```python
from build123d import *

# Parameters (mm, degrees)
Y_KSEKLIK_EKSTR_ZYON1_DEPTH = 7
IZIM2_R                     = 1.5
KES_EKSTR_ZYON1_DEPTH       = 7
PAH1_SIZE                   = 2.5
IZIM3_R                     = 2
KES_EKSTR_ZYON2_DEPTH       = 10
KES_EKSTR_ZYON3_START       = -10
IZIM4_R                     = 2
KES_EKSTR_ZYON3_DEPTH       = 10
RADYUS1_R                   = 20
IZIM5_W                     = 90
IZIM5_H                     = 10
IZIM5_W_2                   = 10
IZIM5_H_2                   = 70
KES_EKSTR_ZYON4_DEPTH       = 10
RADYUS2_R                   = 4
KES_EKSTR_ZYON5_DEPTH       = 10
IZIM8_W                     = 5
IZIM8_H                     = 53
KES_EKSTR_ZYON6_DEPTH       = 10
IZIM9_W                     = 8.724341423
IZIM9_H                     = 2.178581573
IZIM9_W_2                   = 9.164333206
Y_KSEKLIK_EKSTR_ZYON2_DEPTH = 10
IZIM10_W                    = 140
IZIM10_H                    = 10
KES_EKSTR_ZYON7_DEPTH       = 10
IZIM11_W                    = 10
IZIM11_H                    = 4
Y_KSEKLIK_EKSTR_ZYON3_DEPTH = 7
RADYUS3_R                   = 10
IZIM12_W                    = 4
IZIM12_H                    = 9
Y_KSEKLIK_EKSTR_ZYON4_DEPTH = 7
RADYUS4_R                   = 4
IZIM13_R                    = 1.5
KES_EKSTR_ZYON8_DEPTH       = 7
PAH2_SIZE                   = 1.5
RADYUS5_R                   = 2
IZIM14_W                    = 144.535934645
IZIM14_H                    = 70
KES_EKSTR_ZYON9_DEPTH       = 2
RADYUS6_R                   = 2
KES_EKSTR_ZYON10_DEPTH      = 5
KES_EKSTR_ZYON10_DEPTH_BACK = 5
IZIM15_R                    = 7.5
IZIM16_R                    = 1.75
KES_EKSTR_ZYON11_DEPTH      = 7
IZIM17_R                    = 1.75
KES_EKSTR_ZYON12_DEPTH      = 10
Y_KSEKLIK_EKSTR_ZYON5_START = -5
IZIM18_R                    = 3
IZIM18_R_2                  = 2
Y_KSEKLIK_EKSTR_ZYON5_DEPTH = 5
IZIM19_W                    = 4
IZIM19_H                    = 10
KES_EKSTR_ZYON13_DEPTH      = 10


# Some blends are built 0.0001 mm under size
with BuildPart() as part:
    # izim1 → Y_kseklik-Ekstr_zyon1 (new body)
    with BuildSketch(Plane(origin=(0, 0, 0), x_dir=(1, 0, 0), z_dir=(0, 1, 0))):
        Polygon((0, 0), (0, 53), (15, 53), (30, 66.5), (150, 66.5), (150, -13.5), (30, -13.5), (15, 0), align=None)
    extrude(amount=Y_KSEKLIK_EKSTR_ZYON1_DEPTH)

    # izim2 → Kes-Ekstr_zyon1 (cut)
    with BuildSketch(Plane(origin=(0, 7, 0), x_dir=(1, 0, 0), z_dir=(0, 1, 0))):
        with Locations(Location((2.5, 41.25, 0), (0, 0, 270))):
            Circle(IZIM2_R)
        with Locations(Location((2.5, 11.75, 0), (0, 0, 270))):
            Circle(IZIM2_R)
    extrude(amount=-KES_EKSTR_ZYON1_DEPTH, mode=Mode.SUBTRACT)

    # Pah1
    # the kernel refuses this chamfer: 2.5 mm, written as the material it takes off along each edge
    with BuildSketch(Plane(origin=(2.5, 7, -41.25), x_dir=(0, 0, 1), z_dir=(-1, 0, 0))) as pah1_piece_1:
        Polygon((1.5 + PAH1_SIZE, 0), (1.5, -PAH1_SIZE), (1.5, 0), align=None)
    revolve(axis=Axis((2.5, 7, -41.25), (0, 1, 0)), mode=Mode.SUBTRACT)
    with BuildSketch(Plane(origin=(2.5, 7, -11.75), x_dir=(0, 0, 1), z_dir=(-1, 0, 0))) as pah1_piece_2:
        Polygon((1.5 + PAH1_SIZE, 0), (1.5, -PAH1_SIZE), (1.5, 0), align=None)
    revolve(axis=Axis((2.5, 7, -11.75), (0, 1, 0)), mode=Mode.SUBTRACT)

    # izim3 → Kes-Ekstr_zyon2 (cut)
    with BuildSketch(Plane.XY.offset(13.5)):
        with Locations((46.24, 3.5)):
            Circle(IZIM3_R)
    extrude(amount=-KES_EKSTR_ZYON2_DEPTH, mode=Mode.SUBTRACT)

    # izim4 → Kes-Ekstr_zyon3 (cut)
    with BuildSketch(Plane(origin=(0, 0, -66.5), x_dir=(-1, 0, 0), z_dir=(0, 0, -1)).offset(KES_EKSTR_ZYON3_START)):
        with Locations(Location((-46.24, 3.5, 0), (0, 0, 180))):
            Circle(IZIM4_R)
    extrude(amount=KES_EKSTR_ZYON3_DEPTH, mode=Mode.SUBTRACT)

    # Radyus1
    radyus1_edges = [part.edges().sort_by_distance(p)[0] for p in [
        (150, 3.5, -66.5),
        (150, 3.5, 13.5),
    ]]
    fillet(radyus1_edges, radius=RADYUS1_R)

    # izim5 → Kes-Ekstr_zyon4 (cut)
    with BuildSketch(Plane(origin=(0, 7, 0), x_dir=(1, 0, 0), z_dir=(0, 1, 0))):
        with Locations((75, -3.5)):
            Rectangle(IZIM5_W, IZIM5_H)
        with Locations((75, 26.5)):
            Rectangle(IZIM5_W, IZIM5_H)
        with Locations((75, 41.5)):
            Rectangle(IZIM5_W, IZIM5_H)
        with Locations((75, 56.5)):
            Rectangle(IZIM5_W, IZIM5_H)
        with Locations((75, 11.5)):
            Rectangle(IZIM5_W, IZIM5_H)
        with Locations((130, 26.5)):
            Rectangle(IZIM5_W_2, IZIM5_H_2)
    extrude(amount=-KES_EKSTR_ZYON4_DEPTH, mode=Mode.SUBTRACT)

    # Radyus2
    radyus2_edges = [part.edges().sort_by_distance(p)[0] for p in [
        (135, 3.5, -61.5),
        (135, 3.5, 8.5),
    ]]
    fillet(radyus2_edges, radius=RADYUS2_R)

    # izim6 → Kes-Ekstr_zyon5 (cut)
    with BuildSketch(Plane(origin=(0, 7, 0), x_dir=(1, 0, 0), z_dir=(0, 1, 0))):
        with BuildLine():
            Line((139, -6), (139, 59))
            ThreePointArc((139, 59), (143.530979443, 53.484870133), (145, 46.5))
            Line((145, 46.5), (145, 6.5))
            ThreePointArc((145, 6.5), (143.530979443, -0.484870133), (139, -6))
        make_face()
    extrude(amount=-KES_EKSTR_ZYON5_DEPTH, mode=Mode.SUBTRACT)

    # izim8 → Kes-Ekstr_zyon6 (cut)
    with BuildSketch(Plane(origin=(0, 7, 0), x_dir=(1, 0, 0), z_dir=(0, 1, 0))):
        with Locations((2.5, 26.5)):
            Rectangle(IZIM8_W, IZIM8_H)
    extrude(amount=-KES_EKSTR_ZYON6_DEPTH, mode=Mode.SUBTRACT)

    # izim9 → Y_kseklik-Ekstr_zyon2 (add)
    with BuildSketch(Plane.ZY.offset(-5)):
        with Locations((-12.430411948, 5.910709214)):
            Rectangle(IZIM9_W, IZIM9_H)
        with Locations((-41.247168871, 5.910709214)):
            Rectangle(IZIM9_W_2, IZIM9_H)
    extrude(amount=-Y_KSEKLIK_EKSTR_ZYON2_DEPTH)

    # izim10 → Kes-Ekstr_zyon7 (cut)
    with BuildSketch(Plane(origin=(0, 7, 0), x_dir=(1, 0, 0), z_dir=(0, 1, 0))):
        with Locations((85, -13.5)):
            Rectangle(IZIM10_W, IZIM10_H)
        with Locations((85, 66.5)):
            Rectangle(IZIM10_W, IZIM10_H)
    extrude(amount=-KES_EKSTR_ZYON7_DEPTH, mode=Mode.SUBTRACT)


with BuildPart() as kes_ekstr_zyon7_piece_1:
    # of the separate pieces the step leaves, piece 1, a body of its own (kes_ekstr_zyon7_pieces)
    add(part.part.solids().sort_by_distance((24.444444444, 0, 8.5))[0])



with BuildPart() as kes_ekstr_zyon7_piece_2:
    # of the separate pieces the step leaves, piece 2, a body of its own (kes_ekstr_zyon7_pieces)
    add(part.part.solids().sort_by_distance((143.228756555, 0, 8.5))[0])


with BuildPart() as kes_ekstr_zyon7_piece_1_1:
    add(kes_ekstr_zyon7_piece_1.part)

    add(kes_ekstr_zyon7_piece_2.part)  # Y_kseklik-Ekstr_zyon3 merges Kes-Ekstr_zyon7 piece 2
    # izim11 → Y_kseklik-Ekstr_zyon3 (add)
    with BuildSketch(Plane(origin=(0, 7, 0), x_dir=(1, 0, 0), z_dir=(0, 1, 0))):
        with Locations((130, -6.5)):
            Rectangle(IZIM11_W, IZIM11_H)
        with Locations((130, 59.5)):
            Rectangle(IZIM11_W, IZIM11_H)
    extrude(amount=-Y_KSEKLIK_EKSTR_ZYON3_DEPTH)

    # Radyus3
    radyus3_edges = [kes_ekstr_zyon7_piece_1_1.edges().sort_by_distance(p)[0] for p in [
        (120, 3.5, -1.5),
        (120, 3.5, -51.5),
    ]]
    fillet(radyus3_edges, radius=RADYUS3_R - 0.0001)  # a hair under: the kernel refuses the full size

    # izim12 → Y_kseklik-Ekstr_zyon4 (add)
    with BuildSketch(Plane(origin=(0, 7, 0), x_dir=(1, 0, 0), z_dir=(0, 1, 0))):
        with Locations((7, 15)):
            Rectangle(IZIM12_W, IZIM12_H)
        with Locations((7, 38)):
            Rectangle(IZIM12_W, IZIM12_H)
    extrude(amount=Y_KSEKLIK_EKSTR_ZYON4_DEPTH)

    # Radyus4
    radyus4_edges = [kes_ekstr_zyon7_piece_1_1.edges().sort_by_distance(p)[0] for p in [
        (7, 7, -10.5),
        (7, 7, -19.5),
        (7, 7, -33.5),
        (7, 7, -42.5),
    ]]
    fillet(radyus4_edges, radius=RADYUS4_R)

    # izim13 → Kes-Ekstr_zyon8 (cut)
    with BuildSketch(Plane.ZY.offset(-5)):
        with Locations((-38, 10.5)):
            Circle(IZIM13_R)
        with Locations((-15, 10.5)):
            Circle(IZIM13_R)
    extrude(amount=-KES_EKSTR_ZYON8_DEPTH, mode=Mode.SUBTRACT)

    # Pah2
    pah2_edges = [kes_ekstr_zyon7_piece_1_1.edges().sort_by_distance(p)[0] for p in [
        (9, 10.5, -39.5),
        (9, 10.5, -16.5),
    ]]
    chamfer(pah2_edges, length=PAH2_SIZE)

    # Radyus5
    radyus5_edges = [kes_ekstr_zyon7_piece_1_1.edges().sort_by_distance(p)[0] for p in [
        (7, 14, -10.5),
        (7, 14, -19.5),
        (7, 14, -33.5),
        (7, 14, -42.5),
    ]]
    fillet(radyus5_edges, radius=RADYUS5_R)

    # izim14 → Kes-Ekstr_zyon9 (cut)
    with BuildSketch(Plane(origin=(0, 7, 0), x_dir=(1, 0, 0), z_dir=(0, 1, 0))):
        with Locations((81.267967322, 26.5)):
            Rectangle(IZIM14_W, IZIM14_H)
    extrude(amount=-KES_EKSTR_ZYON9_DEPTH, mode=Mode.SUBTRACT)

    # Radyus6
    radyus6_edges = [kes_ekstr_zyon7_piece_1_1.edges().sort_by_distance(p)[0] for p in [
        (7, 7, 0),
        (7, 7, -53),
    ]]
    fillet(radyus6_edges, radius=RADYUS6_R)

    # izim15 → Kes-Ekstr_zyon10 (cut, two sides: drawn at the far end of the back side and taken through both)
    with BuildSketch(Plane(origin=(0, 5, 0), x_dir=(1, 0, 0), z_dir=(0, 1, 0)).offset(-KES_EKSTR_ZYON10_DEPTH_BACK)):
        with Locations((-1, 46.5)):
            Circle(IZIM15_R)
        with Locations((-1, 6.5)):
            Circle(IZIM15_R)
    extrude(amount=KES_EKSTR_ZYON10_DEPTH + KES_EKSTR_ZYON10_DEPTH_BACK, mode=Mode.SUBTRACT)

    # izim16 → Kes-Ekstr_zyon11 (cut)
    with BuildSketch(Plane(origin=(150, 0, 0), x_dir=(0, 0, -1), z_dir=(1, 0, 0))):
        with Locations((26.5, 2.5)):
            Circle(IZIM16_R)
    extrude(amount=-KES_EKSTR_ZYON11_DEPTH, mode=Mode.SUBTRACT)

    # izim17 → Kes-Ekstr_zyon12 (cut)
    with BuildSketch(Plane.XZ):
        with Locations(Location((49, -4, 0), (0, 0, 270))):
            Circle(IZIM17_R)
        with Locations(Location((49, -49, 0), (0, 0, 270))):
            Circle(IZIM17_R)
    extrude(amount=-KES_EKSTR_ZYON12_DEPTH, mode=Mode.SUBTRACT)

    # izim18 → Y_kseklik-Ekstr_zyon5 (add)
    # profile 1 of 2: a face of its own
    with BuildSketch(Plane.XZ.offset(Y_KSEKLIK_EKSTR_ZYON5_START)):
        with Locations((49, -4)):
            Circle(IZIM18_R)
        with Locations((49, -4)):
            Circle(IZIM18_R_2, mode=Mode.SUBTRACT)
    # profile 2 of 2: a face of its own
    with BuildSketch(Plane.XZ.offset(Y_KSEKLIK_EKSTR_ZYON5_START)):
        with Locations((49, -49)):
            Circle(IZIM18_R)
        with Locations((49, -49)):
            Circle(IZIM18_R_2, mode=Mode.SUBTRACT)
    extrude(amount=Y_KSEKLIK_EKSTR_ZYON5_DEPTH)

    # izim19 → Kes-Ekstr_zyon13 (cut)
    with BuildSketch(Plane(origin=(0, 5, 0), x_dir=(1, 0, 0), z_dir=(0, 1, 0))):
        Polygon((22, 51.5), (26, 51.5), (26, 57.5), (22, 53.9), align=None)
        with Locations((24, 41.5)):
            Rectangle(IZIM19_W, IZIM19_H)
        with Locations((24, 26.5)):
            Rectangle(IZIM19_W, IZIM19_H)
        with Locations((24, 11.5)):
            Rectangle(IZIM19_W, IZIM19_H)
        Polygon((22, 1.5), (26, 1.5), (26, -4.5), (22, -0.9), align=None)
        with Locations((16, 41.5)):
            Rectangle(IZIM19_W, IZIM19_H)
        with Locations((16, 26.5)):
            Rectangle(IZIM19_W, IZIM19_H)
        with Locations((16, 11.5)):
            Rectangle(IZIM19_W, IZIM19_H)
    extrude(amount=-KES_EKSTR_ZYON13_DEPTH, mode=Mode.SUBTRACT)


solid = kes_ekstr_zyon7_piece_1_1.part
```
Input: part model. Units: mm. Frame: model coordinates. A direction names the side the tool comes from. Give positions to 0.01 mm unless a question says otherwise; leave off trailing zeros. Order: outer loops, then holes, each group sorted by start corner. A loop starts at its lowest first (then second) coordinate and runs counter-clockwise, first axis right, second up. Notation, with made-up numbers: M 21,57.5 L 78,57.5 A21 cw 78,82.5 Z; hole C 66.5,-6 d1. An arc over 180 degrees is marked long. Return JSON: item names as keys, results as strings.
Item 1: First-contact query: P1, Ø2.5, axis at y = 2.5, z = -52.5, coming from the +X side; P2, Ø3, axis at x = 79, y = 5, coming from the +Z side; P3, Ø8, axis at x = 99, y = 8.5, coming from the -Z side. Flat tips, straight axial feed; report the tip coordinate or a pass-through.
Solutions:
{"P1": "x = 149.43", "P2": "z = -1.5", "P3": "z = -51.5"}
Item 2: Cut plane A-A (x = 81). Return loops of the section in (y, z), then the cut area to 3 significant figures.
Solutions:
{"outline": "M 0,-51.5 L 5,-51.5 L 5,-46.5 L 0,-46.5 Z; M 0,-36.5 L 5,-36.5 L 5,-31.5 L 0,-31.5 Z; M 0,-21.5 L 5,-21.5 L 5,-16.5 L 0,-16.5 Z; M 0,-6.5 L 5,-6.5 L 5,-1.5 L 0,-1.5 Z", "area": "100 mm^2"}
Item 3: Ray query, probe 1 along Z at (x, y) = (85.5, 1); probe 2 along X at (y, z) = (4.5, -56.5); probe 3 along Y at (x, z) = (7, -15). Return the intervals inside material, ascending.
Solutions:
{"probe 1": "-51.5 to -46.5, -36.5 to -31.5, -21.5 to -16.5, -6.5 to -1.5", "probe 2": "18.89 to 24.89, 26 to 30, 118.66 to 125, 135 to 139, 141.61 to 147.32", "probe 3": "0 to 9, 12 to 14"}
Item 4: Cut plane B-B (z = -15). State how many separate pieces and enclosed holes the cut face has, then the cut area to 3 significant figures.
Solutions:
{"separate pieces": "7", "enclosed holes": "0", "area": "177 mm^2"}
Item 5: Access query for faces 1 (the cylindrical face through (7.028, 8.141, -32.297)), 2 (the flat face through (14, 3, -11)), 3 (the cylindrical face through (117.15, 2.46, 1.51)), 4 (the flat face through (39, 3, -51.5)), 5 (the flat face through (131, 3, -61.5)). Directions: +Z, -Z, +X, -X, +Y, -Y. A direction counts if a zero-diameter tool reaches every point of the face in a straight line with its end or side. Return the directions, or none.
Solutions:
{"face 1": "+X, -X, +Y", "face 2": "+Y, -Y", "face 3": "+Z, +Y, -Y", "face 4": "-Z, +Y, -Y", "face 5": "-Z, +X, -X, +Y, -Y"}
Item 6: Cut plane C-C (x = 49). Return loops of the section in (y, z), then the cut area to 3 significant figures.
Solutions:
{"outline": "M 0,-52 L 5,-52 L 5,-50.75 L 0,-50.75 Z; M 0,-47.25 L 5,-47.25 L 5,-46 L 0,-46 Z; M 0,-36.5 L 5,-36.5 L 5,-31.5 L 0,-31.5 Z; M 0,-21.5 L 5,-21.5 L 5,-16.5 L 0,-16.5 Z; M 0,-7 L 5,-7 L 5,-5.75 L 0,-5.75 Z; M 0,-2.25 L 5,-2.25 L 5,-1 L 0,-1 Z", "area": "75.0 mm^2"}
Item 7: Pull-direction query (Z, two-part tool) for faces 6 (the flat face through (5, 6, -26)), 7 (the flat face through (19.656, 2.465, -57.19)), 8 (the flat face through (16, 3, -21.5)), 9 (the flat face through (22, 3, -41)); classes: +Z half, -Z half, draft (parallel to the pull), parting line (faces both ways), or undercut.
Solutions:
{"face 6": "draft", "face 7": "-Z half", "face 8": "undercut", "face 9": "undercut"}
